Could you check a few things on this model? Use its own coordinates, in mm. Round coordinates to 2 decimals unless told otherwise and drop trailing zeros. Write each loop counter-clockwise with the first axis right and the second up, starting at its lowest first coordinate (ties: lowest second). Pieces come first, ordered by that corner, then holes. Notation, with made-up numbers: M -27.75,54.25 L -7.75,54.25 A30 cw -7.75,76.25 Z; hole C 50,-29 d8. An arc over 180 degrees is marked long. One line per item, written item: value. Start each with the question number.
(1) I want a section at D-D on x = 8.5. Please give me the cut outline in (y, z), and give its area (3 significant figures).
(2) If I drill on L1, parallel to Z at x = -15.2, y = 1.4; L2, parallel to X at y = 2.1, z = -8; L3, parallel to Z at x = -23, y = 4.2, over which ranges is the centre line in solid material (lowest first)?
(3) Thinking about a two-plate mould opening in X: for faces 1 (the face through (-7, 3, 0)), 2 (the face through (30, 2, 1)), 3 (the face through (0, 0, -4)), which applies, released by +X, released by -X, zero draft, split by the parting line, or undercut?
(4) I want a section at A-A on x = -15.2. Please give me the cut outline in (y, z).
(5) I want a section at B-B on z = 0. Count the separate pieces of the cut face and the enclosed holes in it, and give its area (4 significant figures).
```python
from build123d import *

# Parameters (mm, degrees)
SKETCH_1_W          = 60
SKETCH_1_H          = 32
EXTRUDE_1_DEPTH     = 5
SKETCH_2_R          = 1.5
SKETCH_2_R_2        = 1.25
SKETCH_2_R_3        = 2.8
CUT_EXTRUDE_1_DEPTH = 5
FILLET_1_R          = 2.5


with BuildPart() as part:
    # 草图1 → 凸台-拉伸1 (new body)
    with BuildSketch(Plane(origin=(0, 0, 0), x_dir=(1, 0, 0), z_dir=(0, 1, 0))):
        Rectangle(SKETCH_1_W, SKETCH_1_H)
    extrude(amount=EXTRUDE_1_DEPTH)

    # 草图2 → 切除-拉伸1 (cut)
    with BuildSketch(Plane(origin=(0, 5, 0), x_dir=(1, 0, 0), z_dir=(0, 1, 0))):
        with Locations(Location((8.5, 0, 0), (0, 0, 270))):
            Circle(SKETCH_2_R)
        with Locations(Location((-8.5, 0, 0), (0, 0, 90))):
            Circle(SKETCH_2_R)
        with Locations(Location((0, 0, 0), (0, 0, 270))):
            Circle(SKETCH_2_R_2)
        with Locations(Location((15.2, 0, 0), (0, 0, 270))):
            Circle(SKETCH_2_R_3)
        with Locations(Location((-15.2, 0, 0), (0, 0, 90))):
            Circle(SKETCH_2_R_3)
        with Locations(Location((15.2, 8, 0), (0, 0, 270))):
            Circle(SKETCH_2_R_2)
        with Locations(Location((23.2, 0, 0), (0, 0, 270))):
            Circle(SKETCH_2_R_2)
        with Locations(Location((-23.2, 0, 0), (0, 0, 90))):
            Circle(SKETCH_2_R_2)
        with Locations(Location((-15.2, 8, 0), (0, 0, 90))):
            Circle(SKETCH_2_R_2)
    extrude(amount=-CUT_EXTRUDE_1_DEPTH, mode=Mode.SUBTRACT)

    # 圆角1
    fillet_1_edges = [part.edges().sort_by_distance(p)[0] for p in [
        (-30, 2.5, -16),
        (30, 2.5, -16),
    ]]
    fillet(fillet_1_edges, radius=FILLET_1_R)


solid = part.part
```
Found:
1. outline: M 0,-16 L 5,-16 L 5,-1.5 L 0,-1.5 Z; M 0,1.5 L 5,1.5 L 5,16 L 0,16 Z
1. area: 145 mm²
2. L1: z = -16 to -9.25, -6.75 to -2.8, 2.8 to 16
2. L2: x = -30 to -16.45, -13.95 to 13.95, 16.45 to 30
2. L3: z = -16 to -1.23, 1.23 to 16
3. face 1: undercut
3. face 2: released by +X
3. face 3: zero draft
4. outline: M 0,-16 L 5,-16 L 5,-9.25 L 0,-9.25 Z; M 0,-6.75 L 5,-6.75 L 5,-2.8 L 0,-2.8 Z; M 0,2.8 L 5,2.8 L 5,16 L 0,16 Z
5. separate pieces: 8
5. enclosed holes: 0
5. area: 176.5 mm²
